Input: dimensioned drawing with shaded views. Units: mm. Origin: part minimum x, y, z. A direction names the side the tool comes from. Round coordinates to 2 decimals unless told otherwise and drop trailing zeros. Order: outer loops, then holes, each group sorted by start corner. A loop starts at its lowest first (then second) coordinate and runs counter-clockwise, first axis right, second up.
Item 1: Line query: L1, parallel to Y at x = 6, z = 2.75; L2, parallel to Y at x = 14.25, z = 5.25; L3, parallel to Z at x = 6, y = 24.5. Output: solid intervals per line, ascending.
Item 2: Cut plane C-C on y = 19. Output: boundary loops of the cut face in (x, z).
Item 3: Reachability of the marked faces 4 and 5 from +Z, -Z, +X, -X, +Y, -Y: full face, straight path, thin tool, end or side. Return the list, or none.
Item 4: Cut plane D-D on x = 9.5. Output: boundary loops of the cut face in (y, z).
Item 5: Mould query, pull axis X, two halves, no side actions, for the marked faces 1, 2 and 3. Classes: released by +X, released by -X, zero draft, split by the parting line, or undercut.
Item 6: Cut plane A-A on z = 7.25. Output: boundary loops of the cut face in (x, y), then the cut area to 3 significant figures.
Item 7: Cut plane B-B on x = 6. Output: boundary loops of the cut face in (y, z), then the cut area to 3 significant figures.
Item 8: First-contact query: pin 1 (5 mm diameter, centred on y = 25, z = 2.5, fed in from +X); pin 2 (11 mm diameter, centred on x = 14, y = 17.5, fed in from +Z). Flat tips, straight axial feed; report the tip coordinate or a pass-through.
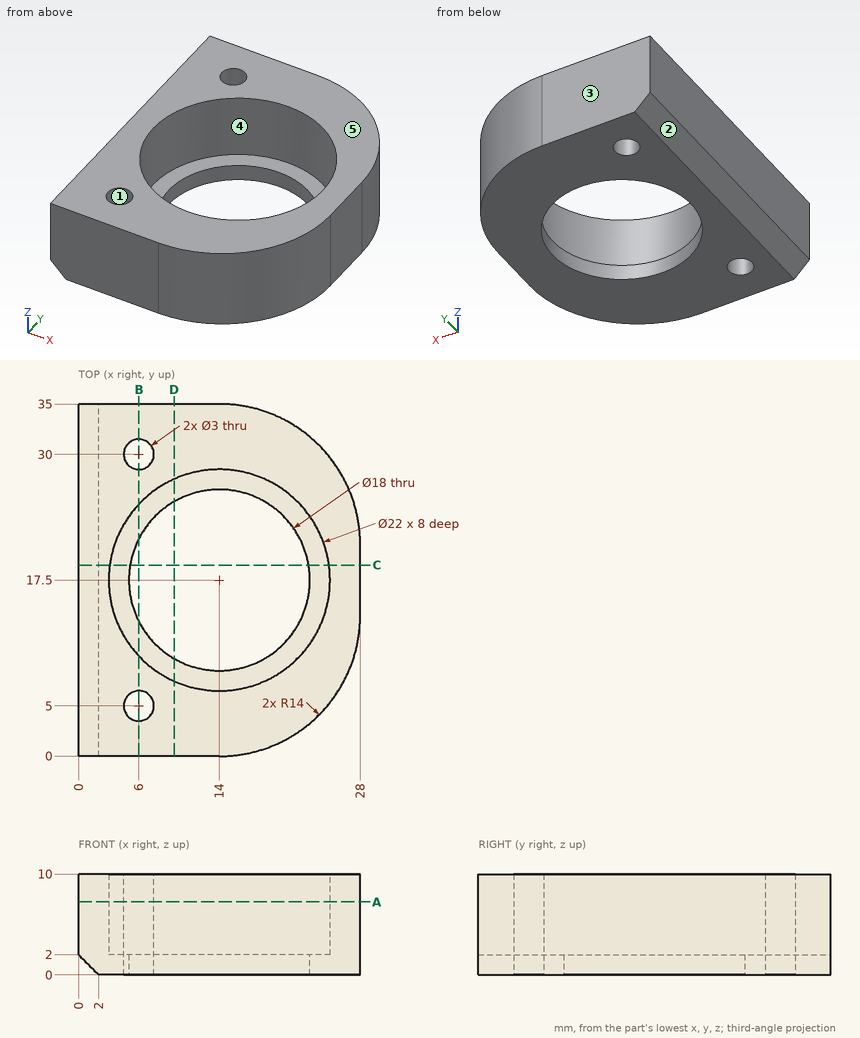
From the geometry:
1. L1: y = 0 to 3.5, 6.5 to 9.95, 25.05 to 28.5, 31.5 to 35
1. L2: y = 0 to 6.5, 28.5 to 35
1. L3: z = 0 to 2
2. outline: (0, 2) - (2, 0) - (5.13, 0) - (5.13, 2) - (3.1, 2) - (3.1, 10) - (0, 10) - close; (22.87, 0) - (28, 0) - (28, 10) - (24.9, 10) - (24.9, 2) - (22.87, 2) - close
3. face 4: +Z
3. face 5: +Z, +X, -X, +Y, -Y
4. outline: (0, 0) - (9.71, 0) - (9.71, 2) - (7.46, 2) - (7.46, 10) - (0, 10) - close; (25.29, 0) - (35, 0) - (35, 10) - (27.54, 10) - (27.54, 2) - (25.29, 2) - close
5. face 1: undercut
5. face 2: released by -X
5. face 3: zero draft
6. outline: (0, 0) - (14, 0) arc R14 ccw to (28, 14) - (28, 21) arc R14 ccw to (14, 35) - (0, 35) - close; hole circle Ø22 at (14, 17.5); hole circle Ø3 at (6, 5); hole circle Ø3 at (6, 30)
6. area: 502 mm2
7. outline: (0, 0) - (3.5, 0) - (3.5, 10) - (0, 10) - close; (6.5, 0) - (13.38, 0) - (13.38, 2) - (9.95, 2) - (9.95, 10) - (6.5, 10) - close; (21.62, 0) - (28.5, 0) - (28.5, 10) - (25.05, 10) - (25.05, 2) - (21.62, 2) - close; (31.5, 0) - (35, 0) - (35, 10) - (31.5, 10) - close
7. area: 153 mm2
8. pin 1: stops at x = 27.92
8. pin 2: passes through
